from build123d import *

# Parameters (mm, degrees)
SCHIZZO1_R                   = 5.5
ESTRUSIONE_ESTRUSIONE1_DEPTH = 2.9
SCHIZZO2_R                   = 3.9
ESTRUSIONE_ESTRUSIONE2_DEPTH = 5
SCHIZZO3_R                   = 4
ESTRUSIONE_ESTRUSIONE3_DEPTH = 7
SCHIZZO4_R                   = 3
TAGLIO_ESTRUSIONE1_DEPTH     = 10
SCHIZZO5_W                   = 3
SCHIZZO5_H                   = 9.5
ESTRUSIONE_ESTRUSIONE4_DEPTH = 0.4
SCHIZZO7_W                   = 3
SCHIZZO7_H                   = 6
ESTRUSIONE_ESTRUSIONE5_DEPTH = 0.4
SCHIZZO8_W                   = 3
SCHIZZO8_H                   = 6
ESTRUSIONE_ESTRUSIONE6_DEPTH = 0.4


with BuildPart() as part:
    # Schizzo1 → Estrusione-Estrusione1 (new body)
    with BuildSketch(Plane(origin=(0, 0, 0), x_dir=(1, 0, 0), z_dir=(0, 1, 0))):
        with Locations(Location((0, 0, 0), (0, 0, 270))):
            Circle(SCHIZZO1_R)
    extrude(amount=ESTRUSIONE_ESTRUSIONE1_DEPTH)

    # Schizzo2 → Estrusione-Estrusione2 (add)
    with BuildSketch(Plane(origin=(0, 2.9, 0), x_dir=(1, 0, 0), z_dir=(0, 1, 0))):
        with Locations(Location((0, 0, 0), (0, 0, 270))):
            Circle(SCHIZZO2_R)
    extrude(amount=ESTRUSIONE_ESTRUSIONE2_DEPTH)

    # Schizzo3 → Estrusione-Estrusione3 (add)
    with BuildSketch(Plane.XZ):
        with Locations(Location((0, 0, 0), (0, 0, 270))):
            Circle(SCHIZZO3_R)
    extrude(amount=ESTRUSIONE_ESTRUSIONE3_DEPTH)

    # Schizzo4 → Taglio-Estrusione1 (cut)
    with BuildSketch(Plane(origin=(0, 7.9, 0), x_dir=(1, 0, 0), z_dir=(0, 1, 0))):
        with Locations(Location((0, 0, 0), (0, 0, 270))):
            Circle(SCHIZZO4_R)
    extrude(amount=-TAGLIO_ESTRUSIONE1_DEPTH, mode=Mode.SUBTRACT)

    # Schizzo5 → Estrusione-Estrusione4 (add)
    with BuildSketch(Plane.XY.offset(3.8)):
        with Locations((0, -7.75)):
            Rectangle(SCHIZZO5_W, SCHIZZO5_H)
    extrude(amount=ESTRUSIONE_ESTRUSIONE4_DEPTH)

    # Schizzo7 → Estrusione-Estrusione5 (add)
    with BuildSketch(Plane(origin=(-3.8, 0, 0), x_dir=(0, 0, -1), z_dir=(1, 0, 0))):
        with Locations((0, -9.5)):
            Rectangle(SCHIZZO7_W, SCHIZZO7_H)
    extrude(amount=-ESTRUSIONE_ESTRUSIONE5_DEPTH)

    # Schizzo8 → Estrusione-Estrusione6 (add)
    with BuildSketch(Plane.XY.offset(-3.8)):
        with Locations((0, -9.5)):
            Rectangle(SCHIZZO8_W, SCHIZZO8_H)
    extrude(amount=-ESTRUSIONE_ESTRUSIONE6_DEPTH)


solid = part.part
Build history of the part. All positions in model axes, mm. A direction names the side the tool comes from. Round coordinates to 2 decimals unless told otherwise and drop trailing zeros. Write each loop counter-clockwise with the first axis right and the second up, starting at its lowest first coordinate (ties: lowest second). Pieces come first, ordered by that corner, then holes. Notation, with made-up numbers: (-27, 21) - (22, 21) arc R30 cw to (22, 47) - close; hole circle Ø7 at (-38, 28.25). An arc over 180 degrees is marked (long way). Use CSV: the item, a comma, the result in double quotes.
(1) Wall check: line 1 (X direction, y = 0.25, z = 0); line 2 (Y direction, x = -2.25, z = -2.5); line 3 (Y direction, x = -4.25, z = -2.25). Give the ranges that are in metal, low to high.
Response:
line 1,"-5.5 to -3, 3 to 5.5"
line 2,"-7 to 7.9"
line 3,"0 to 2.9"
(2) Band-saw the part on A-A (y = -10). Write the cut outline in (x, z).
Response:
outline,"(-4.2, -1.5) - (-3.8, -1.5) - (-3.8, 1.5) - (-4.2, 1.5) - close; (-1.5, -4.2) - (1.5, -4.2) - (1.5, -3.8) - (-1.5, -3.8) - close; (-1.5, 3.8) - (1.5, 3.8) - (1.5, 4.2) - (-1.5, 4.2) - close"
(3) Pin check, flat tips, straight feed: P1, Ø0.9, axis at x = -0.5, y = -9.5, coming from the -Z side; P2, Ø1, axis at y = 2.5, z = -2, coming from the +X side; P3, Ø2, axis at x = -3, y = -2.5, coming from the -Z side. Stop position of each tip, or through.
Response:
P1,"z = -4.2"
P2,"x = 5.29"
P3,"z = -3.46"
(4) 3-axis set-ups, long thin cutter, end or side, ignore diameter. For faces 4 (the cylindrical face through (1.201, -3.451, -3.815)), 5 (the flat face through (-4.2, -9, 0)), 6 (the flat face through (0, -2.1, 0)), 7 (the flat face through (0, -7, 0)): which of +Z, -Z, +X, -X, +Y, -Y reach the whole face in a straight line?
Response:
face 4,"none"
face 5,"+Z, -Z, -X, -Y"
face 6,"+Y"
face 7,"+X, -Y"
(5) Mould opens along Z. For faces 1 (the flat face through (0, -9, -4.2)), 2 (the cylindrical face through (0.9, 2.97, 2.86)), 3 (the flat face through (4, 2.9, 1)) say: pulls with the +Z half, pulls with the -Z half, needs draft (parallel to the pull), parting line crosses it, or undercut.
Response:
face 1,"pulls with the -Z half"
face 2,"undercut"
face 3,"needs draft"
(6) Band-saw the part on D-D (y = 0.5). Write the cut outline in (x, z).
Response:
outline,"circle Ø11 at (0, 0); hole circle Ø6 at (0, 0)"
(7) Band-saw the part on B-B (x = 0). Write the cut outline in (y, z).
Response:
outline,"(-12.5, -4.2) - (-6.5, -4.2) - (-6.5, -4) - (0, -4) - (0, -5.5) - (2.9, -5.5) - (2.9, -3.9) - (7.9, -3.9) - (7.9, -3) - (-2.1, -3) - (-2.1, 3) - (7.9, 3) - (7.9, 3.9) - (2.9, 3.9) - (2.9, 5.5) - (0, 5.5) - (0, 4) - (-3, 4) - (-3, 4.2) - (-12.5, 4.2) - (-12.5, 3.8) - (-7, 3.8) - (-7, -3.8) - (-12.5, -3.8) - close"
(8) Band-saw the part on C-C (z = 0). Write the cut outline in (x, y).
Response:
outline,"(-5.5, 0) - (-4, 0) - (-4, -6.5) - (-4.2, -6.5) - (-4.2, -12.5) - (-3.8, -12.5) - (-3.8, -7) - (4, -7) - (4, 0) - (5.5, 0) - (5.5, 2.9) - (3.9, 2.9) - (3.9, 7.9) - (3, 7.9) - (3, -2.1) - (-3, -2.1) - (-3, 7.9) - (-3.9, 7.9) - (-3.9, 2.9) - (-5.5, 2.9) - close"
